from build123d import *

# Parameters (mm, degrees)
SKETCH1_W                 = 6
SKETCH1_H                 = 40
BOSS_EXTRUDE1_DEPTH       = 5
SKETCH3_R                 = 1.5
CUT_EXTRUDE1_DEPTH        = 41.755367745
LPATTERN1_COUNT           = 4
LPATTERN1_PITCH           = 10
BOSS_EXTRUDE3_DEPTH       = 6
SKETCH12_R                = 1.5
BOSS_EXTRUDE7_DEPTH       = 8
SKETCH10_W                = 20
SKETCH10_H                = 5
BOSS_EXTRUDE6_DEPTH       = 15
CUT_EXTRUDE2_REACH        = 50.278
SKETCH11_R                = 5
FILLET1_R                 = 10
BOSS_EXTRUDE8_START       = -20.169777786
BOSS_EXTRUDE8_OUTLINE_R   = 3
BOSS_EXTRUDE8_OUTLINE_R_2 = 1.5
BOSS_EXTRUDE8_DEPTH       = 4


# Read off the part's stored shape, not the designer's step: Boss-Extrude8
with BuildPart() as part:
    # Sketch1 → Boss-Extrude1 (new body)
    with BuildSketch(Plane(origin=(0, 0, 0), x_dir=(1, 0, 0), z_dir=(0, 1, 0))):
        with Locations((3, 20)):
            Rectangle(SKETCH1_W, SKETCH1_H)
    extrude(amount=BOSS_EXTRUDE1_DEPTH)

    # Sketch3 → Cut-Extrude1 (cut, through all)
    with BuildSketch(Plane(origin=(0, 0, 0), x_dir=(1, 0, 0), z_dir=(0, 1, 0))):
        with Locations(Location((3, 6, 0), (0, 0, 270))):
            Circle(SKETCH3_R)
    cut_extrude1 = extrude(amount=CUT_EXTRUDE1_DEPTH, mode=Mode.SUBTRACT)

    # LPattern1: Cut-Extrude1 ×4
    with Locations(*[(0, 0, -i * LPATTERN1_PITCH) for i in range(1, LPATTERN1_COUNT)]):
        add(cut_extrude1, mode=Mode.SUBTRACT)

    # Sketch4 → Boss-Extrude3 (add)
    with BuildSketch(Plane(origin=(0, 0, 0), x_dir=(0, 0, -1), z_dir=(1, 0, 0))):
        Polygon((-11.570176974, -8.788799976), (-7.739954759, -12.002738025), (3.830222216, 1.786061952), (0, 5), align=None)
    extrude(amount=BOSS_EXTRUDE3_DEPTH)

    # Sketch12 → Boss-Extrude7 (add)
    with BuildSketch(Plane(origin=(0, -10.854679532, 9.108157592), x_dir=(1, 0, 0), z_dir=(0, -0.7660444431189747, 0.6427876096865434))):
        with Locations(Location((3, 0.713938048, 0), (0, 0, 90))):
            Circle(SKETCH12_R)
    extrude(amount=BOSS_EXTRUDE7_DEPTH)

    # Sketch10 → Boss-Extrude6 (add)
    with BuildSketch(Plane.ZY):
        with Locations((-30, 2.5)):
            Rectangle(SKETCH10_W, SKETCH10_H)
    extrude(amount=BOSS_EXTRUDE6_DEPTH)

    # Sketch11 → Cut-Extrude2 (cut, up to next)
    with BuildSketch(Plane(origin=(0, 5, 0), x_dir=(1, 0, 0), z_dir=(0, 1, 0)), mode=Mode.PRIVATE) as cut_extrude2_sk1:
        with Locations(Location((-7, 30, 0), (0, 0, 270))):
            Circle(SKETCH11_R)
    cut_extrude2_tool1 = extrude(cut_extrude2_sk1.sketch, amount=-CUT_EXTRUDE2_REACH, mode=Mode.PRIVATE) & part.part
    add(cut_extrude2_tool1.solids().sort_by_distance((-7, 5, -30))[0], mode=Mode.SUBTRACT)

    # Fillet1
    fillet1_edges = [part.edges().sort_by_distance(p)[0] for p in [
        (-15, 2.5, -40),
        (-15, 2.5, -20),
    ]]
    fillet(fillet1_edges, radius=FILLET1_R - 0.0001)  # a hair under: the kernel refuses the full size

    # Boss-Extrude8 outline → Boss-Extrude8 (add)
    with BuildSketch(Plane(origin=(0, 0, 0), x_dir=(1, 0, 0), z_dir=(0, 0.766044443118975, -0.642787609686543)).offset(BOSS_EXTRUDE8_START)):
        with Locations((3, -0.713938048)):
            Circle(BOSS_EXTRUDE8_OUTLINE_R)
        with Locations((3, -0.713938048)):
            Circle(BOSS_EXTRUDE8_OUTLINE_R_2, mode=Mode.SUBTRACT)
    extrude(amount=BOSS_EXTRUDE8_DEPTH)


solid = part.part
Build history of the part. All positions in model axes, mm. A direction names the side the tool comes from. Round coordinates to 2 decimals unless told otherwise and drop trailing zeros. Write each loop counter-clockwise with the first axis right and the second up, starting at its lowest first coordinate (ties: lowest second). Pieces come first, ordered by that corner, then holes. Notation, with made-up numbers: M 17,39 L 56,39 A12 ccw 56,54 Z; hole C 28.25,81.5 d5. An arc over 180 degrees is marked long. Answer as a JSON object with one key per item and string values. Group by question number.
(1) Drill centre lines: L1, parallel to Z at x = 3, y = 3.9; L2, parallel to Z at x = 3, y = 1.7; L3, parallel to X at y = 3.1, z = -6. Where is each one in solid material? Low to high.
(2) Mould opens along Y. For faces 1 (the flat face through (2.96, -9.3, 10.96)), 2 (the cylindrical face through (2.1, 2.5, -37.2)), 3 (the flat face through (-2, 5, -25)) say: pulls with the +Y half, pulls with the -Y half, needs draft (parallel to the pull), parting line crosses it, or undercut.
(3) Cut at B-B (x = -2.75). Give the cut face in (y, z).
(4) Flat gauge pins, fed straight in: pin 1 (4 mm diameter, centred on x = -1.5, y = 3, fed in from +Z); pin 2 (2.5 mm diameter, centred on x = 3, z = -36, fed in from -Y); pin 3 (4 mm diameter, centred on x = 3, z = -6, fed in from -Y); pin 4 (8.5 mm diameter, centred on y = -5.5, z = -2.5, fed in from -X). Where does each tip first touch, or does it go through?
(5) Which spindle directions (+Z, -Z, +X, -X, +Y, -Y) get a long thin tool onto all of the face, cutting with end or side? Do faces 4 (the flat face through (0, 0, -2)), 5 (the flat face through (4.29, -11.1, 11.93)), 6 (the flat face through (-2, 0, -26)), 7 (the cylindrical face through (2.1, 2.5, -7.2)). Say none if no direction does.
(6) Cut at A-A (z = -16). Give the cut face in (x, y), and give its area (3 significant figures).
(7) Cut at C-C (y = 1.25). Give the number of separate pieces and of enclosed holes in the cut face, and give its area (3 significant figures).
Responses:
{
 "1": {"L1": "z = -40 to -37.5, -34.5 to -27.5, -24.5 to -17.5, -14.5 to -7.5, -4.5 to 0.92", "L2": "z = -40 to -37.5, -34.5 to -27.5, -24.5 to -17.5, -14.5 to -7.5, -4.5 to 2.77", "L3": "x = 0 to 1.5, 4.5 to 6"},
 "2": {"face 1": "undercut", "face 2": "needs draft", "face 3": "pulls with the +Y half"},
 "3": {"outline": "M 0,-40 L 5,-40 L 5,-32.63 L 0,-32.63 Z; M 0,-27.37 L 5,-27.37 L 5,-20 L 0,-20 Z"},
 "4": {"pin 1": "stops at z = 2.79", "pin 2": "passes through", "pin 3": "stops at y = 0", "pin 4": "stops at x = 0"},
 "5": {"face 4": "+Z, -X, +Y, -Y", "face 5": "none", "face 6": "-Z, +X, -X, -Y", "face 7": "+Y, -Y"},
 "6": {"outline": "M 0,0 L 1.5,0 L 1.5,5 L 0,5 Z; M 4.5,0 L 6,0 L 6,5 L 4.5,5 Z", "area": "15.0 mm2"},
 "7": {"separate pieces": "1", "enclosed holes": "5", "area": "409 mm2"}
}
